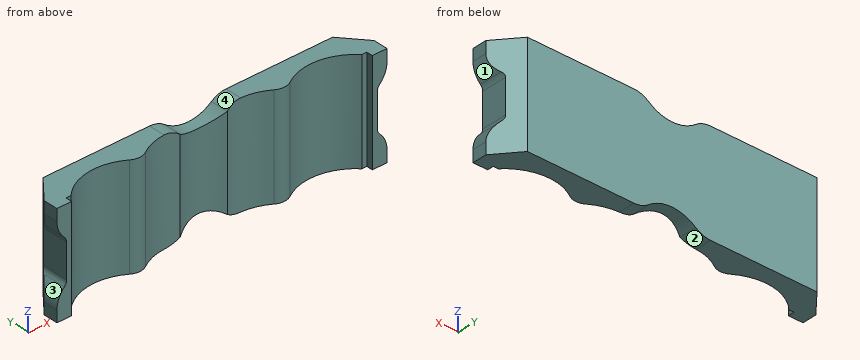
from build123d import *
from OCP.BRepFilletAPI import BRepFilletAPI_MakeChamfer

# Parameters (mm, degrees)
BOSS_EXTRUDE2_DEPTH = 21.2
CHAMFER1_SIZE       = 5
CHAMFER1_SIZE2      = 4.195498156
CUT_EXTRUDE1_DEPTH  = 42.067048835
FILLET2_R           = 5
FILLET3_R           = 3
CUT_EXTRUDE2_DEPTH  = 42.067048989
FILLET4_R           = 5
CUT_EXTRUDE3_DEPTH  = 42.067048989


with BuildPart() as part:
    # Sketch4 → Boss-Extrude2 (new body)
    with BuildSketch(Plane.XY):
        with BuildLine():
            Line((-34.25, 0), (34.25, 0))
            Line((34.25, 0), (34.25, -8))
            Line((34.25, -8), (31.2, -8))
            Line((31.2, -8), (31.2, -6.7))
            Line((31.2, -6.7), (30.2, -6.7))
            ThreePointArc((30.2, -6.7), (22.642993845, -3.400961512), (15, -6.49557652))
            ThreePointArc((15, -6.49557652), (7.5, -3.4), (0, -6.49557652))
            ThreePointArc((0, -6.49557652), (-7.5, -3.4), (-15, -6.49557652))
            ThreePointArc((-15, -6.49557652), (-22.642993845, -3.400961512), (-30.2, -6.7))
            Line((-30.2, -6.7), (-31.2, -6.7))
            Line((-31.2, -6.7), (-31.2, -8))
            Line((-31.2, -8), (-34.25, -8))
            Line((-34.25, -8), (-34.25, 0))
        make_face()
    extrude(amount=BOSS_EXTRUDE2_DEPTH)

    # Chamfer1: one chamfer whose edges measure the first distance from different faces: ONE call of the kernel's chamfer builder (chamfer() names one face for all edges)
    chamfer1_edges_1 = [part.edges().sort_by_distance(p)[0] for p in [
        (-34.25, 0, 10.6),
    ]]
    chamfer1_side_1 = [part.faces().sort_by_distance(p)[0] for p in [
        (-34.25, -4, 10.6),
    ]]
    chamfer1_edges_2 = [part.edges().sort_by_distance(p)[0] for p in [
        (34.25, 0, 10.6),
    ]]
    chamfer1_side_2 = [part.faces().sort_by_distance(p)[0] for p in [
        (34.25, -4, 10.6),
    ]]
    chamfer1 = BRepFilletAPI_MakeChamfer(part.part.solid().wrapped)
    for e in chamfer1_edges_1:
        chamfer1.Add(CHAMFER1_SIZE, CHAMFER1_SIZE2, e.wrapped, chamfer1_side_1[0].wrapped)  # the first distance lies on this face
    for e in chamfer1_edges_2:
        chamfer1.Add(CHAMFER1_SIZE, CHAMFER1_SIZE2, e.wrapped, chamfer1_side_2[0].wrapped)  # the first distance lies on this face
    add(Compound.cast(chamfer1.Shape()), mode=Mode.REPLACE)

    # Sketch5 → Cut-Extrude1 (cut, through all)
    with BuildSketch(Plane(origin=(0, 0, 0), x_dir=(1, 0, 0), z_dir=(0, 1, 0))):
        with BuildLine():
            Line((-6, 0), (6, 0))
            ThreePointArc((6, 0), (0, -2.708497378), (-6, 0))
        make_face()
        with BuildLine():
            Line((-6, -21.2), (6, -21.2))
            ThreePointArc((6, -21.2), (0, -18.491502622), (-6, -21.2))
        make_face()
    extrude(amount=-CUT_EXTRUDE1_DEPTH, mode=Mode.SUBTRACT)

    # Fillet2
    fillet2_edges = [part.edges().sort_by_distance(p)[0] for p in [
        (6, -1.753165508, 21.2),
        (-6, -1.753165508, 21.2),
        (-6, -1.753165508, 0),
        (6, -1.753165508, 0),
    ]]
    fillet(fillet2_edges, radius=FILLET2_R)

    # Fillet3
    fillet3_edges = [part.edges().sort_by_distance(p)[0] for p in [
        (-15, -6.49557652, 10.6),
        (0, -6.49557652, 10.6),
        (15, -6.49557652, 10.6),
    ]]
    fillet(fillet3_edges, radius=FILLET3_R)

    # Sketch6 → Cut-Extrude2 (cut, through all)
    with BuildSketch(Plane(origin=(0, 0, 0), x_dir=(1, 0, 0), z_dir=(0, 1, 0))):
        with BuildLine():
            Line((34.25, -5.6), (33.75, -5.6))
            ThreePointArc((33.75, -5.6), (32.689339828, -6.039339828), (32.25, -7.1))
            Line((32.25, -7.1), (32.25, -14.1))
            ThreePointArc((32.25, -14.1), (32.689339828, -15.160660172), (33.75, -15.6))
            Line((33.75, -15.6), (34.25, -15.6))
            Line((34.25, -15.6), (34.25, -5.6))
        make_face()
        with BuildLine():
            Line((-32.25, -7.1), (-32.25, -14.1))
            ThreePointArc((-32.25, -14.1), (-32.689339828, -15.160660172), (-33.75, -15.6))
            Line((-33.75, -15.6), (-34.25, -15.6))
            Line((-34.25, -15.6), (-34.25, -5.6))
            Line((-34.25, -5.6), (-33.75, -5.6))
            ThreePointArc((-33.75, -5.6), (-32.689339828, -6.039339828), (-32.25, -7.1))
        make_face()
    extrude(amount=-CUT_EXTRUDE2_DEPTH, mode=Mode.SUBTRACT)

    # Fillet4
    # the kernel refuses this fillet: 5 mm, written as the material it takes off along each edge
    with BuildSketch(Plane(origin=(-34.25, 2.9760394, 15.6), x_dir=(0, 0, 1), z_dir=(0, -1, 0)), Plane(origin=(34.25, 2.9760394, 5.6), x_dir=(0, 0, -1), z_dir=(0, -1, 0))) as fillet4_piece_1:
        with BuildLine():
            CenterArc((3.19041576, -5), FILLET4_R, 90, 46.18693854)
            Line((-0.417596363, -1.538461538), (-0.778397575, -1.192307692))
            ThreePointArc((-0.778397575, -1.192307692), (-0.5, -0.5), (-0.5, 0))
            Line((-0.5, 0), (0, 0.5))
            Line((0, 0.5), (3.19041576, 0.5))
            Line((3.19041576, 0.5), (3.19041576, 0))
        make_face()
    extrude(amount=18.952078799, mode=Mode.SUBTRACT)
    with BuildSketch(Plane(origin=(-34.25, 2.9760394, 5.6), x_dir=(0, 0, -1), z_dir=(0, -1, 0)), Plane(origin=(34.25, 2.9760394, 15.6), x_dir=(0, 0, 1), z_dir=(0, -1, 0))) as fillet4_piece_2:
        with BuildLine():
            CenterArc((3.19041576, 5), FILLET4_R, 223.81306146, 46.18693854)
            Line((-0.417596363, 1.538461538), (-0.778397575, 1.192307692))
            ThreePointArc((-0.778397575, 1.192307692), (-0.5, 0.5), (-0.5, 0))
            Line((-0.5, 0), (0, -0.5))
            Line((0, -0.5), (3.19041576, -0.5))
            Line((3.19041576, -0.5), (3.19041576, 0))
        make_face()
    extrude(amount=18.952078799, mode=Mode.SUBTRACT)

    # Sketch7 → Cut-Extrude3 (cut, through all)
    with BuildSketch(Plane.XY):
        with BuildLine():
            ThreePointArc((-4.887756907, -3.725862072), (0, -2.449957006), (4.887756907, -3.725862072))
            ThreePointArc((4.887756907, -3.725862072), (3.209259906, -4.304133612), (1.650366748, -5.153605376))
            ThreePointArc((1.650366748, -5.153605376), (0, -5.648352974), (-1.650366748, -5.153605376))
            ThreePointArc((-1.650366748, -5.153605376), (-3.209259906, -4.304133612), (-4.887756907, -3.725862072))
        make_face()
    extrude(amount=CUT_EXTRUDE3_DEPTH, mode=Mode.SUBTRACT)


solid = part.part
Could you check a few things on this model? Use its own coordinates, in mm. Face numbers are marked on the shaded views. A direction names the side the tool comes from. Coordinates: 2 decimals unless noted, no trailing zeros. Loops run counter-clockwise (first coordinate to the right, second up) from the corner with the lowest first, then second, coordinate; pieces in that order, holes last. Notation, with made-up numbers: (28.25, 6) -> (50.25, 6) arc R32 ccw to (50.25, 44) -> close; hole circle Ø2 at (-12, 37). An arc over 180 degrees is marked (long way). Answer in a Markdown table with one row per item.
(1) If I drill on probe 1 along X at (y, z) = (-6.75, 3.5); probe 2 along Y at (x, z) = (-23, 6.5); probe 3 along X at (y, z) = (-6.5, 8), over which ranges is the centre line in solid material (lowest first)?
Results found:
| item | result |
|---|---|
| probe 1 | x = -34.13 to -31.2, 31.2 to 34.13 |
| probe 2 | y = -3.41 to 0 |
| probe 3 | x = -32.25 to -30, 30 to 32.25 |
(2) Imagine slicing it at B-B (x = 28). List the corners of the cut face in (y, z) for me, plus the area to 3 significant figures.
Results found:
| item | result |
|---|---|
| outline | (-4.93, 0) -> (0, 0) -> (0, 21.2) -> (-4.93, 21.2) -> close |
| area | 105 mm^2 |
(3) Will these pins go through, and if not, where does the flat tip stop? pin 1 Ø3 at (y, z) = (-5, 16) entering from -X; pin 2 Ø4.5 at (y, z) = (-4, 11) entering from +X; pin 3 Ø0.8 at (x, z) = (-31, 10) entering from -Y; pin 4 Ø1 at (x, z) = (-16, 8) entering from -Y.
Results found:
| item | result |
|---|---|
| pin 1 | stops at x = -34.08 |
| pin 2 | stops at x = 32.25 |
| pin 3 | stops at y = -8 |
| pin 4 | stops at y = -5.61 |
(4) For the marked faces 1, 2, 3 and 4, which set-ups out of +Z, -Z, +X, -X, +Y, -Y let a thin tool reach every point of the face, with its end or its side?
Results found:
| item | result |
|---|---|
| face 1 | +X, +Y, -Y |
| face 2 | -Z, +Y, -Y |
| face 3 | -X, +Y, -Y |
| face 4 | +Z, +Y, -Y |
(5) Imagine slicing it at C-C (x = -10). List the corners of the cut face in (y, z) for me, plus the area to 3 significant figures.
Results found:
| item | result |
|---|---|
| outline | (-3.7, 0) -> (0, 0) -> (0, 21.2) -> (-3.7, 21.2) -> close |
| area | 78.4 mm^2 |
(6) Imagine slicing it at A-A (y = -1.5). List the corners of the cut face in (x, z) for me.
Results found:
| item | result |
|---|---|
| outline | (-31.31, 0) -> (-7.94, 0) arc R5 ccw to (-4.89, 1.04) arc R8 cw to (4.89, 1.04) arc R5 ccw to (7.94, 0) -> (31.31, 0) -> (31.31, 21.2) -> (7.94, 21.2) arc R5 ccw to (4.89, 20.16) arc R8 cw to (-4.89, 20.16) arc R5 ccw to (-7.94, 21.2) -> (-31.31, 21.2) -> close |
